CAD build for the part. Positions are in the model's coordinates, mm. A direction names the side the tool comes from. Coordinates: 2 decimals unless noted, no trailing zeros. Order: outer loops, then holes, each group sorted by start corner. A loop starts at its lowest first (then second) coordinate and runs counter-clockwise, first axis right, second up. Notation, with made-up numbers: (52, 48) -> (66, 48) arc R24 ccw to (66, 84) -> close; hole circle Ø3 at (1.25, 45). An arc over 180 degrees is marked (long way). Use one line per item in the form item = value. Start each with the question number.
from build123d import *

# Parameters (mm, degrees)
F0_W           = 175
F0_H           = 135
F1_DEPTH       = 75
F2_W           = 12.7
F2_H           = 20
F3_DEPTH       = 92.1
F5_D           = 22
F5_DEPTH       = 180
F5_CBORE_D     = 33
F5_CBORE_DEPTH = 30


with BuildPart() as f1:
    # F0 (on Front) → F1 (new body)
    with BuildSketch(Plane.XZ):
        with Locations((-87.5, 67.5)):
            Rectangle(F0_W, F0_H)
    extrude(amount=F1_DEPTH)

    # F2 (on face) → F3 (cut)
    with BuildSketch(Plane.XZ.offset(75)):
        with Locations((-93.85, 0)):
            Rectangle(F2_W, F2_H)
        with Locations((-81.15, 0)):
            Rectangle(F2_W, F2_H)
    extrude(amount=-F3_DEPTH, mode=Mode.SUBTRACT)

    # F5
    with Locations(Plane.XY.offset(135)):
        with Locations((-87.5, -37.5)):
            CounterBoreHole(F5_D / 2, F5_CBORE_D / 2, F5_CBORE_DEPTH, depth=F5_DEPTH)


solid = f1.part
1) Probe L1, parallel to X at y = -37, z = 76; L2, parallel to Y at x = -87.5, z = 82; L3, parallel to Y at x = -87.5, z = 120.75. List the from-to ranges inside material, lowest first.
2) Cut at C-C on z = 28. Give the cut face in (x, y), then the cut area to 3 significant figures.
3) Cut at B-B on y = -37.5. Give the cut face in (x, z).
4) Two-plate mould, pull along X, no slides. Class faces 4 (the face through (-91.077, -53.608, 120.21)), 5 (the face through (-100.2, -38, 5)), 6 (the face through (-89, -75, 68)), 7 (the face through (-175, -37, 67)): released by +X, released by -X, zero draft, split by the parting line, or undercut.
5) 3-axis set-ups, long thin cutter, end or side, ignore diameter. For faces 1 (the face through (-76.51, -37.02, 56.84)), 2 (the face through (-74.8, -38, 5)), 3 (the face through (-76.7, -40.9, 105)): which of +Z, -Z, +X, -X, +Y, -Y reach the whole face in a straight line?
6) Cut at A-A on x = -87.5. Give the cut face in (y, z).
Values follow:
q1.L1 = -175 to -98.49, -76.51 to 0
q1.L2 = -75 to -48.5, -26.5 to 0
q1.L3 = -75 to -54, -21 to 0
q2.outline = (-175, -75) -> (0, -75) -> (0, 0) -> (-175, 0) -> close; hole circle Ø22 at (-87.5, -37.5)
q2.area = 12,700 mm^2
q3.outline = (-175, 0) -> (-100.2, 0) -> (-100.2, 10) -> (-98.5, 10) -> (-98.5, 105) -> (-104, 105) -> (-104, 135) -> (-175, 135) -> close; (-76.5, 10) -> (-74.8, 10) -> (-74.8, 0) -> (0, 0) -> (0, 135) -> (-71, 135) -> (-71, 105) -> (-76.5, 105) -> close
q4.face_4 = undercut
q4.face_5 = undercut
q4.face_6 = zero draft
q4.face_7 = released by -X
q5.face_1 = +Z, -Z
q5.face_2 = -Z, +Y, -Y
q5.face_3 = +Z
q6.outline = (-75, 10) -> (-48.5, 10) -> (-48.5, 105) -> (-54, 105) -> (-54, 135) -> (-75, 135) -> close; (-26.5, 10) -> (0, 10) -> (0, 135) -> (-21, 135) -> (-21, 105) -> (-26.5, 105) -> close
